Design review of the part built by this model. Coordinates are the model's own, in mm. A direction names the side the tool comes from. Coordinates: 2 decimals unless noted, no trailing zeros.
Q1. Add section A-A, the plane z = 12. Give the number of separate pieces and of enclosed holes in the cut face, plus the area to 3 significant figures.
Q2. To check wall thickness, follow probe 1 along Y at (x, z) = (91.5, 15.5); probe 2 along Y at (x, z) = (92.25, 14.5); probe 3 along Z at (x, y) = (92, -23.5). State the ranges of each line that lie inside material, in increasing order.
Q3. Clearance check with flat-ended pins moving along their axes: pin 1 Ø6 at (x, z) = (89.5, 21) entering from -Y; pin 2 Ø4.5 at (x, y) = (87.5, -25) entering from +Z; pin 3 Ø3 at (x, y) = (94, 23.5) entering from -Z; pin 4 Ø2 at (x, y) = (82.5, 5) entering from +Z. State where each tip first meets the part, or that it passes through.
Q4. The part is to be moulded in two halves that separate along Z. For faces 5 (the face through (87.4, 10.07, 12.71)), 6 (the face through (90.133, 48.643, 37.049)), 7 (the face through (83, 42, 31)), 8 (the face through (90.133, -30.427, 17.292)), say which applies: +Z half, -Z half, draft (parallel to the pull), parting line (faces both ways), or undercut.
Q5. Machinability: for faces 1 (the face through (82.7, -22, 18)), 2 (the face through (97, 0, 16)), 3 (the face through (99.246, 51.573, 6.479)), 4 (the face through (81.689, 0.132, 18.824)), which of the approach directions +Z, -Z, +X, -X, +Y, -Y give a long, thin tool a straight path to every point of the face, cutting with its end or side? Answer none if there is none.
from build123d import *

# Parameters (mm, degrees)
PAD016_DEPTH      = 9.5
POCKET008_DEPTH   = 7
POCKET009_DEPTH   = 7.3
PAD017_DEPTH      = 4.1
PAD017_DEPTH_BACK = 9.5
PAD018_DEPTH      = 9.5
SKETCH031_R       = 2.1
PAD019_DEPTH      = 3


with BuildPart() as part:
    # Sketch026 → Pad016 (new body, symmetric)
    with BuildSketch(Plane.YZ):
        Polygon((47.4801846947, 33.7107123063), (39.698240274, 28.2617361609), (31.9162958532, 22.8127600156), (29.7273220428, 21.6732523754), (20.8002421453, 18.4240610138), (11.8731622478, 15.1748696522), (9.4638496319, 14.6407379046), (0, 13.8127583485), (-9.4638496319, 12.9847787924), (-11.9293103801, 13.0924231333), (-21.2849840337, 14.7420808212), (-30.6406576873, 16.391738509), (-31.335250398, 12.452507497), (-12.6239030908, 9.1531921213), (-9.1152266609, 9), (9.8124726029, 10.6559591122), (13.2412428211, 11.416099169), (31.0954026161, 17.9144818922), (34.2106015986, 19.5361518385), (49.7744904401, 30.4341041291), align=None)
    extrude(amount=PAD016_DEPTH, both=True)

    # Sketch027 → Pocket008 (cut, symmetric)
    with BuildSketch(Plane.YZ):
        Polygon((-28.1786383048, 15.9576180648), (-21.2849840337, 14.7420808212), (-14.3913297626, 13.5265435775), (-14.6344372114, 12.1478127233), (-13.3541871324, 11.9220700923), (-13.8056723944, 9.3615699345), (-21.9795767444, 10.8028498091), (-30.1534810944, 12.2441296838), (-29.7019958324, 14.8046298416), (-28.4217457535, 14.5788872106), align=None)
        Polygon((-6.9733628866, 13.2026681492), (0, 13.8127583485), (6.9733628866, 14.4228485477), (7.0953809265, 13.0281759704), (8.390434034, 13.1414784359), (8.6170389652, 10.5513722209), (0.348622971, 9.8279795561), (-7.9197930232, 9.1045868913), (-8.1463979543, 11.6946931063), (-6.8513448468, 11.8079955719), align=None)
        Polygon((14.2223937998, 16.0299200105), (20.8002421453, 18.4240610138), (27.3780904908, 20.818202017), (27.8569186914, 19.5026323479), (29.0785190985, 19.9472585343), (29.9677714711, 17.5040577202), (22.1683227186, 14.6652905306), (14.3688739661, 11.826523341), (13.4796215934, 14.2697241551), (14.7012220004, 14.7143503414), align=None)
        Polygon((33.964175964, 24.2467011065), (39.698240274, 28.2617361609), (45.432304584, 32.2767712154), (46.2353115949, 31.1299583534), (47.3002092525, 31.8756077207), (48.791507987, 29.7458124055), (41.9925460194, 24.9851279838), (35.1935840518, 20.2244435621), (33.7022853173, 22.3542388772), (34.7671829748, 23.0998882445), align=None)
    extrude(amount=POCKET008_DEPTH, both=True, mode=Mode.SUBTRACT)

    # Sketch028 → Pocket009 (cut, symmetric)
    with BuildSketch(Plane.YZ):
        Polygon((-28.387016118, 14.7758487612), (-14.5997075758, 12.3447742739), (-14.6344372114, 12.1478127233), (-13.3541871324, 11.9220700923), (-13.4931056746, 11.1342238899), (-29.8409143746, 14.0167836392), (-29.7019958324, 14.8046298416), (-28.4217457535, 14.5788872106), align=None)
        Polygon((-6.8687759953, 12.0072345115), (7.0779497779, 13.22741491), (7.0953809265, 13.0281759704), (8.390434034, 13.1414784359), (8.4601586282, 12.3445226775), (-8.0766733601, 10.8977373479), (-8.1463979543, 11.6946931063), (-6.8513448468, 11.8079955719), align=None)
        Polygon((14.6328179718, 14.9022888655), (27.7885146628, 19.6905708721), (27.8569186914, 19.5026323479), (29.0785190985, 19.9472585343), (29.3521352131, 19.1955044376), (13.7532377081, 13.5179700584), (13.4796215934, 14.2697241551), (14.7012220004, 14.7143503414), align=None)
        Polygon((34.6524676876, 23.2637186533), (46.1205963076, 31.2937887623), (46.2353115949, 31.1299583534), (47.3002092525, 31.8756077207), (47.7590704016, 31.2202860852), (34.1611464664, 21.6989172418), (33.7022853173, 22.3542388772), (34.7671829748, 23.0998882445), align=None)
    extrude(amount=POCKET009_DEPTH, both=True, mode=Mode.SUBTRACT)

    # Sketch029 → Pad017 (join, two sides)
    with BuildSketch(Plane.YZ) as pad017_sk:
        Polygon((9.4638496319, 14.6407379046), (9.8124726029, 10.6559591122), (10.3354070593, 4.6787909237), (10.3354070593, 0), (15.2933636811, 0), (15.2933636811, 5.7779434443), (13.2412428211, 11.416099169), (11.8731622478, 15.1748696522), align=None)
    extrude(amount=PAD017_DEPTH)
    extrude(pad017_sk.sketch, amount=-PAD017_DEPTH_BACK)

    # Sketch030 → Pad018 (join)
    with BuildSketch(Plane.YZ):
        with BuildLine():
            Line((-13.6657921568, 3.2443456032), (-12.6239030908, 9.1531921213))
            Line((-12.6239030908, 9.1531921213), (-11.9293103801, 13.0924231333))
            Line((-11.9293103801, 13.0924231333), (-9.4638496319, 12.9847787924))
            Line((-9.4638496319, 12.9847787924), (-9.1152266609, 9))
            Line((-9.1152266609, 9), (-8.5922922044, 3.0228318114))
            Line((-8.5922922044, 3.0228318114), (-15, 0))
            Line((-15, 0), (-25, 0))
            Line((-25, 0), (-25, 3))
            add(Edge.make_bspline(
                [(-13.6657921568, 3.2443456032), (-13.9496356176, 1.6345893441), (-20, 3), (-25, 3)],
                knots=[0, 0, 0, 0, 1, 1, 1, 1], degree=3))
        make_face()
        with BuildLine():
            Line((37.6520602167, 14.6212395727), (34.2106015986, 19.5361518385))
            Line((34.2106015986, 19.5361518385), (31.9162958532, 22.8127600156))
            Line((31.9162958532, 22.8127600156), (29.7273220428, 21.6732523754))
            Line((29.7273220428, 21.6732523754), (31.0954026161, 17.9144818922))
            Line((31.0954026161, 17.9144818922), (33.147523476, 12.2763261675))
            Line((33.147523476, 12.2763261675), (35, 0))
            Line((35, 0), (45, 0))
            Line((45, 0), (45, 3))
            add(Edge.make_bspline(
                [(37.6520602167, 14.6212395727), (42.2621193459, 8.0373928164), (40, 3), (45, 3)],
                knots=[0, 0, 0, 0, 1, 1, 1, 1], degree=3))
        make_face()
    extrude(amount=-PAD018_DEPTH)

    # Sketch031 → Pad019 (join)
    with BuildSketch(Plane.XY):
        with BuildLine():
            Line((7.6224992299, -26.0948753465), (0, -20))
            Line((0, -20), (0, -25))
            Line((0, -25), (-9.5, -25))
            Line((-9.5, -25), (-9.5, -35))
            Line((-9.5, -35), (4.5, -35))
            ThreePointArc((4.5, -35), (9.218348401, -31.6544450327), (7.6224992299, -26.0948753465))
        make_face()
        with Locations((0, -30)):
            Circle(SKETCH031_R, mode=Mode.SUBTRACT)
        with BuildLine():
            Line((0, 45), (-9.5, 45))
            Line((-9.5, 45), (-9.5, 55))
            Line((-9.5, 55), (4.5, 55))
            ThreePointArc((7.6224992299, 46.0948753465), (9.218348401, 51.6544450327), (4.5, 55))
            Line((7.6224992299, 46.0948753465), (0, 40))
            Line((0, 40), (0, 45))
        make_face()
        with Locations((0, 50)):
            Circle(SKETCH031_R, mode=Mode.SUBTRACT)
    extrude(amount=PAD019_DEPTH)


with BuildPart() as part_1:
    # Body004 placement: moved
    add(part.part.moved(Location((90, 0, 5))))


solid = part_1.part
Here are the results:
1. separate pieces: 3
1. enclosed holes: 0
1. area: 170 mm2
2. probe 1: y = -13.6 to -8.04, 9.83 to 13.57
2. probe 2: y = -13.78 to -7.95, 9.91 to 13.94
2. probe 3: z = 5 to 8
3. pin 1: stops at y = -31.24
3. pin 2: stops at z = 8
3. pin 3: passes through
3. pin 4: stops at z = 19.34
4. face 5: -Z half
4. face 6: +Z half
4. face 7: undercut
4. face 8: undercut
5. face 1: none
5. face 2: -Z
5. face 3: -Z, +X
5. face 4: +Z, +X, -X
